Source: CAD feature listing. Evaluate the final solid. Frame: model axes, mm. Face numbers are marked on the shaded views. A direction names the side the tool comes from. Coordinates: 2 decimals unless noted, no trailing zeros. Order: outer loops, then holes, each group sorted by start corner. A loop starts at its lowest first (then second) coordinate and runs counter-clockwise, first axis right, second up.
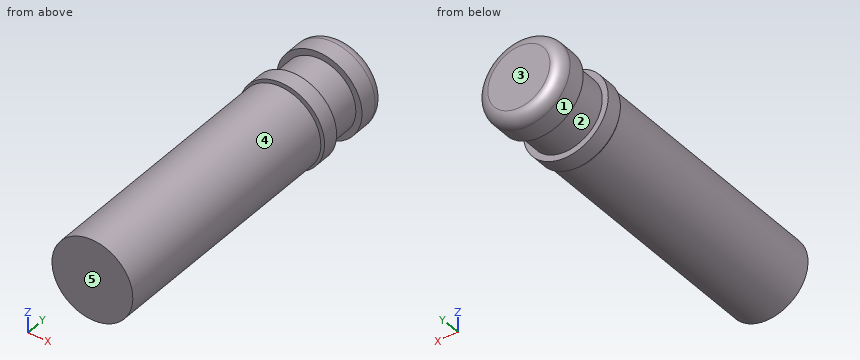
```python
from build123d import *


with BuildPart() as part:
    # 草图1 → 旋转4 (revolve)
    with BuildSketch(Plane(origin=(0, 0, 0), x_dir=(0, 0, -1), z_dir=(1, 0, 0)), mode=Mode.PRIVATE) as revolve_4_sk:
        with BuildLine():
            Line((-7, 0), (0, 0))
            Line((0, 0), (0, 58))
            Line((0, 58), (-5.378171024, 58))
            ThreePointArc((-5.378171024, 58), (-6.792384586, 57.414213562), (-7.378171024, 56))
            Line((-7.378171024, 56), (-7.378171024, 52.933330123))
            Line((-7.378171024, 52.933330123), (-6.309364611, 52.933330123))
            Line((-6.309364611, 52.933330123), (-6.309364611, 47.048318533))
            Line((-6.309364611, 47.048318533), (-7.354829453, 47.048318533))
            Line((-7.354829453, 47.048318533), (-7.354829453, 44.220608725))
            Line((-7.354829453, 44.220608725), (-6.309364611, 44.220608725))
            Line((-6.309364611, 44.220608725), (-6.309364611, 43.835644878))
            Line((-6.309364611, 43.835644878), (-7, 43.835644878))
            Line((-7, 43.835644878), (-7, 0))
        make_face()
    revolve(revolve_4_sk.sketch.rotate(Axis((0, 0, 0), (0, 1, 0)), 180), axis=Axis((0, 0, 0), (0, 1, 0)))


solid = part.part
```
Q1. Section query D-D on y = 28.5. Output: boundary loops of the cut face in (x, z), plus the area to 3 significant figures.
Solutions:
outline: circle Ø14 at (0, 0)
area: 154 mm2
Q2. Section query C-C on y = 49. Output: boundary loops of the cut face in (x, z).
Solutions:
outline: circle Ø12.62 at (0, 0)
Q3. Section query B-B on z = 0. Output: boundary loops of the cut face in (x, y).
Solutions:
outline: (-7.38, 52.93) - (-6.31, 52.93) - (-6.31, 47.05) - (-7.35, 47.05) - (-7.35, 44.22) - (-6.31, 44.22) - (-6.31, 43.84) - (-7, 43.84) - (-7, 0) - (7, 0) - (7, 43.84) - (6.31, 43.84) - (6.31, 44.22) - (7.35, 44.22) - (7.35, 47.05) - (6.31, 47.05) - (6.31, 52.93) - (7.38, 52.93) - (7.38, 56) arc R2 ccw to (5.38, 58) - (-5.38, 58) arc R2 ccw to (-7.38, 56) - close
Q4. Pin query (flat end, axial travel): P1, Ø4, axis at x = 1, y = 8, coming from the -Z side; P2, Ø3, axis at x = 2.5, y = 50, coming from the -Z side; P3, Ø1, axis at x = -5.5, y = 37.5, coming from the +Z side. Return the tip coordinate at first contact, or that it passes through.
Solutions:
P1: stops at z = -7
P2: stops at z = -6.23
P3: stops at z = 4.9
Q5. Pull-direction query (Y, two-part tool) for the marked faces 1, 2 and 3; classes: pulls with the +Y half, pulls with the -Y half, needs draft (parallel to the pull), parting line crosses it, or undercut.
Solutions:
face 1: needs draft
face 2: undercut
face 3: pulls with the +Y half
Q6. Set-up query: the marked faces 4 and 5. Return all of +Z, -Z, +X, -X, +Y, -Y with unobstructed straight access to the full face (end or side cutting, diameter ignored); none if empty.
Solutions:
face 4: -Y
face 5: +Z, -Z, +X, -X, -Y
Q7. Material intervals for line 1 along Y through (x, z) = (1.5, 6.25); line 2 along Y through (x, z) = (3.5, -5.5); line 3 along Y through (x, z) = (-5.5, -0.25), sorted ascending.
Solutions:
line 1: y = 0 to 43.84, 44.22 to 47.05, 52.93 to 57.7
line 2: y = 0 to 43.84, 44.22 to 47.05, 52.93 to 57.64
line 3: y = 0 to 58
Q8. Section query A-A on x = 0. Output: boundary loops of the cut face in (y, z).
Solutions:
outline: (0, -7) - (43.84, -7) - (43.84, -6.31) - (44.22, -6.31) - (44.22, -7.35) - (47.05, -7.35) - (47.05, -6.31) - (52.93, -6.31) - (52.93, -7.38) - (56, -7.38) arc R2 ccw to (58, -5.38) - (58, 5.38) arc R2 ccw to (56, 7.38) - (52.93, 7.38) - (52.93, 6.31) - (47.05, 6.31) - (47.05, 7.35) - (44.22, 7.35) - (44.22, 6.31) - (43.84, 6.31) - (43.84, 7) - (0, 7) - close
